```python
from build123d import *

# Parameters (mm, degrees)
SKETCH_1_R      = 39.5
SKETCH_1_R_2    = 10
EXTRUDE_1_DEPTH = 3
FILLET_1_R      = 20
FILLET_2_R      = 20


with BuildPart() as part:
    # Эскиз1 → Бобышка-Вытянуть1 (new body)
    with BuildSketch(Plane.XY):
        with BuildLine():
            Line((-73.038609064, 50.411192066), (-50.411192066, 73.038609064))
            Line((-50.411192066, 73.038609064), (-21.285640845, 110.360884799))
            ThreePointArc((-21.285640845, 110.360884799), (0, 120.75), (21.285640845, 110.360884799))
            Line((21.285640845, 110.360884799), (50.411192066, 73.038609064))
            Line((50.411192066, 73.038609064), (73.038609064, 50.411192066))
            ThreePointArc((73.038609064, 50.411192066), (132.287319575, -38.537319575), (43.338807934, 20.711390936))
            Line((43.338807934, 20.711390936), (23.534235961, 40.515962909))
            ThreePointArc((23.534235961, 40.515962909), (0, 26.75), (-23.534235961, 40.515962909))
            Line((-23.534235961, 40.515962909), (-43.338807934, 20.711390936))
            ThreePointArc((-43.338807934, 20.711390936), (-132.287319575, -38.537319575), (-73.038609064, 50.411192066))
        make_face()
        with Locations((-93.75, 0)):
            Circle(SKETCH_1_R, mode=Mode.SUBTRACT)
        with Locations((93.75, 0)):
            Circle(SKETCH_1_R, mode=Mode.SUBTRACT)
        with Locations((0, 53.75)):
            Circle(SKETCH_1_R_2, mode=Mode.SUBTRACT)
    extrude(amount=EXTRUDE_1_DEPTH)

    # Скругление1
    fillet_1_edges = [part.edges().sort_by_distance(p)[0] for p in [
        (23.534235961, 40.515962909, 1.5),
        (-23.534235961, 40.515962909, 1.5),
    ]]
    fillet(fillet_1_edges, radius=FILLET_1_R)

    # Скругление2
    # the kernel refuses this fillet: 20 mm, written as the material it adds along each edge
    with BuildSketch(Plane(origin=(73.038609064, 50.411192066, 0), x_dir=(0.9564465824657693, 0.29190740807583243, 0), z_dir=(0, 0, 1))) as fillet_2_piece_1:
        with BuildLine():
            CenterArc((12.057212621, 19.912448006), FILLET_2_R, 208.027815678, 56.6091051)
            Line((-5.59717882, 10.514444874), (-5.950266649, 10.326484811))
            Line((-5.950266649, 10.326484811), (-0.353087829, -0.187960063))
            Line((-0.353087829, -0.187960063), (0.037386706, -0.39824896))
            ThreePointArc((0.037386706, -0.39824896), (5.093938665, -0.161420815), (10.150490625, -0.39824896))
            Line((10.150490625, -0.39824896), (10.187877331, 0))
        make_face()
    extrude(amount=3)
    with BuildSketch(Plane(origin=(-73.038609064, 50.411192066, 0), x_dir=(-0.9564465824657701, 0.2919074080758299, 0), z_dir=(0, 0, 1))) as fillet_2_piece_2:
        with BuildLine():
            CenterArc((12.057212621, -19.912448006), FILLET_2_R, 95.363079222, 56.6091051)
            Line((-5.59717882, -10.514444874), (-5.950266649, -10.326484811))
            Line((-5.950266649, -10.326484811), (-0.353087829, 0.187960063))
            Line((-0.353087829, 0.187960063), (0.037386706, 0.39824896))
            ThreePointArc((0.037386706, 0.39824896), (5.093938665, 0.161420815), (10.150490625, 0.39824896))
            Line((10.150490625, 0.39824896), (10.187877331, 0))
        make_face()
    extrude(amount=3)
    with BuildSketch(Plane(origin=(43.338807934, 20.711390936, 0), x_dir=(-0.7071067811865486, 0.7071067811865466, 0), z_dir=(0, 0, 1))) as fillet_2_piece_3:
        with BuildLine():
            CenterArc((12.095099349, 19.719973869), FILLET_2_R, 213.13333953, 47.267573146)
            Line((-4.652916781, 8.788187386), (-4.987877104, 8.569551657))
            ThreePointArc((-4.987877104, 8.569551657), (-2.479115111, 4.313269402), (-0.369110171, -0.154135272))
            Line((-0.369110171, -0.154135272), (0, -0.4))
            ThreePointArc((0, -0.4), (4.380019269, -0.4), (8.693337321, -0.394399477))
            Line((8.693337321, -0.394399477), (8.760038538, 0))
        make_face()
    extrude(amount=3)
    with BuildSketch(Plane(origin=(-43.338807934, 20.711390936, 0), x_dir=(0.7071067811865474, 0.7071067811865477, 0), z_dir=(0, 0, 1))) as fillet_2_piece_4:
        with BuildLine():
            CenterArc((12.095099349, -19.719973869), FILLET_2_R, 99.599087325, 47.267573146)
            Line((-4.652916781, -8.788187386), (-4.987877104, -8.569551657))
            ThreePointArc((-4.987877104, -8.569551657), (-2.479115111, -4.313269402), (-0.369110171, 0.154135272))
            Line((-0.369110171, 0.154135272), (0, 0.4))
            ThreePointArc((0, 0.4), (4.380019269, 0.4), (8.693337321, 0.394399477))
            Line((8.693337321, 0.394399477), (8.760038538, 0))
        make_face()
    extrude(amount=3)


solid = part.part
```
Here's how the part is built. I have some questions about the finished solid (model axes, mm). Coordinates: 2 decimals unless noted, no trailing zeros. Loops run counter-clockwise (first coordinate to the right, second up) from the corner with the lowest first, then second, coordinate; pieces in that order, holes last. Notation, with made-up numbers: (49, -3) - (89, -3) arc R8 cw to (89, 4) - close; hole circle Ø4 at (76.5, 11). An arc over 180 degrees is marked (long way). Return JSON: item names as keys, results as strings. Group by question number.
Item 1: Will these pins go through, and if not, where does the flat tip stop? P1, Ø1, axis at x = -5.5, z = 1, coming from the +Y side; P2, Ø1.5, axis at y = 63, z = 1.5, coming from the +X side.
Item 2: If we section it at A-A on x = -93.75: Write out the boundary of the cut face in (y, z).
Item 3: We'd pull the mould along Y, two halves only. Please class faces 1 (the face through (54.29, 1.74, 1.48)), 2 (the face through (25.55, 32.6, 1.52)), 3 (the face through (-73.15, 53.78, 1.48)): +Y half, -Y half, draft (parallel to the pull), parting line (faces both ways), or undercut.
Item 4: If we section it at B-B on y = 0: Write out the boundary of the cut face in (x, z), and give its area (3 significant figures).
Item 5: If we section it at D-D on x = 100: Write out the boundary of the cut face in (y, z), and give its area (3 significant figures).
Item 6: I need wall thicknesses on line 1 (Y direction, x = 93.75, z = 1.5); line 2 (X direction, y = 16, z = 2.9); line 3 (X direction, y = 22.5, z = 0.25). Which ranges of each line are inside material? Lowest first, please. Write a range as from..to.
Item 7: If we section it at C-C on z = 1.45: Write out the boundary of the cut face in (x, y).
Calculated:
{
 "1": {"P1": "stops at y = 120.28", "P2": "stops at x = 61.2"},
 "2": {"outline": "(-54.5, 0) - (-39.5, 0) - (-39.5, 3) - (-54.5, 3) - close; (39.5, 0) - (54.5, 0) - (54.5, 3) - (39.5, 3) - close"},
 "3": {"face 1": "undercut", "face 2": "-Y half", "face 3": "+Y half"},
 "4": {"outline": "(-148.25, 0) - (-133.25, 0) - (-133.25, 3) - (-148.25, 3) - close; (-54.25, 0) - (-39.25, 0) - (-39.25, 3) - (-54.25, 3) - close; (39.25, 0) - (54.25, 0) - (54.25, 3) - (39.25, 3) - close; (133.25, 0) - (148.25, 0) - (148.25, 3) - (133.25, 3) - close", "area": "180 mm^2"},
 "5": {"outline": "(-54.14, 0) - (-39, 0) - (-39, 3) - (-54.14, 3) - close; (39, 0) - (54.14, 0) - (54.14, 3) - (39, 3) - close", "area": "90.8 mm^2"},
 "6": {"line 1": "y = -54.5..-39.5, 39.5..54.5", "line 2": "x = -145.85..-129.86, -57.64..-40.83, 40.83..57.64, 129.86..145.85", "line 3": "x = -143.39..-126.22, -61.28..-39.51, 39.51..61.28, 126.22..143.39"},
 "7": {"outline": "(-82.78, 53.39) arc R54.5 ccw (long way) to (-40.41, 11.21) arc R20 cw to (-37.14, 26.91) arc R20 cw to (-13.21, 30.2) arc R27 ccw to (13.21, 30.2) arc R20 cw to (37.14, 26.91) arc R20 cw to (40.41, 11.21) arc R54.5 ccw (long way) to (82.78, 53.39) arc R20 cw to (64.62, 58.83) - (50.41, 73.04) - (21.29, 110.36) arc R27 ccw to (-21.29, 110.36) - (-50.41, 73.04) - (-64.62, 58.83) arc R20 cw to start; hole circle Ø79 at (-93.75, 0); hole circle Ø20 at (0, 53.75); hole circle Ø79 at (93.75, 0)"}
}
